Could you check a few things on this drawing? It's one solid part, dimensions in mm from its lowest x, y, z. A direction names the side the tool comes from. Give positions to 0.01 mm unless a question says otherwise; leave off trailing zeros. Order: outer loops, then holes, each group sorted by start corner. A loop starts at its lowest first (then second) coordinate and runs counter-clockwise, first axis right, second up.
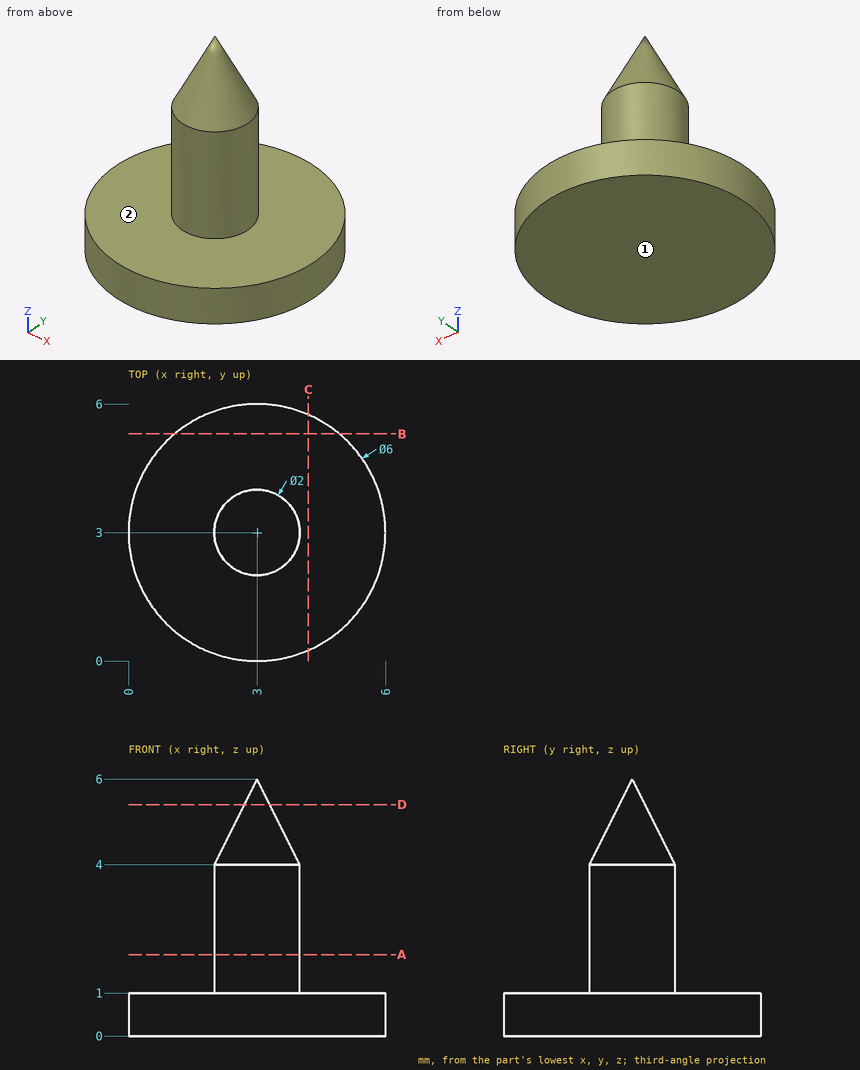
Item 1: Imagine slicing it at B-B on y = 5.3. List the corners of the cut face in (x, z) for me, then the cut area to 3 significant figures.
Findings:
outline: (1.07, 0) - (4.93, 0) - (4.93, 1) - (1.07, 1) - close
area: 3.85 mm2
Item 2: For the marked faces 1 and 2, which set-ups out of +Z, -Z, +X, -X, +Y, -Y let a thin tool reach every point of the face, with its end or its side?
Findings:
face 1: -Z, +X, -X, +Y, -Y
face 2: +Z
Item 3: Imagine slicing it at C-C on x = 4.2. List the corners of the cut face in (y, z) for me.
Findings:
outline: (0.25, 0) - (5.75, 0) - (5.75, 1) - (0.25, 1) - close
Item 4: Imagine slicing it at D-D on z = 5.4. List the corners of the cut face in (x, y) for me, then the cut area to 3 significant figures.
Findings:
outline: circle Ø0.6 at (3, 3)
area: 0.283 mm2
Item 5: For pin 1 (1.5 mm diameter, centred on y = 3, z = 3.5, fed in from -X); pin 2 (1.5 mm diameter, centred on x = 4, z = 1, fed in from +Y); pin 3 (1 mm diameter, centred on x = 4, z = 4, fed in from -Y); pin 4 (2 mm diameter, centred on x = 2.5, y = 2.5, fed in from +Z), each with a flat end and sliding along its axis, tell me the tip position at first contact or that it passes through.
Findings:
pin 1: stops at x = 2
pin 2: stops at y = 5.99
pin 3: stops at y = 2.13
pin 4: stops at z = 6
Item 6: Imagine slicing it at A-A on z = 1.9. List the corners of the cut face in (x, y) for me.
Findings:
outline: circle Ø2 at (3, 3)
Item 7: Please list where these lines run through material, in increasing order: line 1 along Z through (x, y) = (4.2, 0.85); line 2 along X through (y, z) = (2.6, 2.2); line 3 along Y through (x, z) = (2.35, 2.7).
Findings:
line 1: z = 0 to 1
line 2: x = 2.08 to 3.92
line 3: y = 2.24 to 3.76
